Work out the finished part from the listing and answer in its coordinate system (mm). A direction names the side the tool comes from. Give positions to 0.01 mm unless a question says otherwise; leave off trailing zeros. Write each loop counter-clockwise with the first axis right and the second up, starting at its lowest first coordinate (ties: lowest second). Pieces come first, ordered by that corner, then holes. Notation, with made-up numbers: (28, -38.75) - (44, -38.75) arc R27 ccw to (44, -9.75) - close; hole circle Ø1 at (28, -24). An arc over 180 degrees is marked (long way). Write item = value, one per line.
from build123d import *

# Parameters (mm, degrees)
F0_W     = 64
F0_H     = 80
F0_W_2   = 1
F1_DEPTH = 10
F2_T     = -2
F3_DEPTH = 8
F5_DEPTH = 130.001
F6_START = -25.25
F4_R     = 1
F6_DEPTH = 27.25
F8_W     = 1.5
F8_H     = 2
F9_DEPTH = 2.4
F10_R    = 5
F11_R    = 3


# Not quite as in the source:
# - a pattern or mirror of a feature is missing from the dataset's text; its kind, count and spacing are read off the source's solid


with BuildPart() as f1:
    # F0 (on Top) → F1 (new body)
    with BuildSketch(Plane.XY):
        with Locations((-32, 40)):
            Rectangle(F0_W, F0_H)
        with Locations((-64.5, 40)):
            Rectangle(F0_W_2, F0_H)
        with Locations((-65.5, 40)):
            Rectangle(F0_W_2, F0_H)
        with Locations((-98, 40)):
            Rectangle(F0_W, F0_H)
    extrude(amount=F1_DEPTH)

    # F2
    f2_openings = [f1.faces().sort_by_distance(p)[0] for p in [
        (-65, 40, 10),
    ]]
    offset(amount=F2_T, openings=f2_openings)

    # F0 (on Top) → F3 (join)
    with BuildSketch(Plane.XY):
        with Locations((-65.5, 40)):
            Rectangle(F0_W_2, F0_H)
        with Locations((-64.5, 40)):
            Rectangle(F0_W_2, F0_H)
    extrude(amount=F3_DEPTH)

    # F4 (on face) → F5 (cut, through all)
    with BuildSketch(Plane.YZ):
        with BuildLine():
            ThreePointArc((0, 7.8458905733), (0.7245313434, 8.5770948967), (0.9894327009, 9.5717972144))
            ThreePointArc((0.9894327009, 9.5717972144), (0.9778046189, 9.7871506811), (0.9430555853, 10))
            Line((0.9430555853, 10), (0.840551923, 10))
            ThreePointArc((0.840551923, 10), (0.8771729534, 9.7872890681), (0.8894327009, 9.5717972144))
            ThreePointArc((0.8894327009, 9.5717972144), (0.6522733229, 8.6525795765), (0, 7.9628367631))
            Line((0, 7.9628367631), (0, 7.8458905733))
        make_face()
        with BuildLine():
            ThreePointArc((0.8894327009, 9.5717972144), (0.8771729534, 9.7872890681), (0.840551923, 10))
            Line((0.840551923, 10), (0, 10))
            Line((0, 10), (0, 7.9628367631))
            ThreePointArc((0, 7.9628367631), (0.6522733229, 8.6525795765), (0.8894327009, 9.5717972144))
        make_face()
    extrude(amount=-F5_DEPTH, mode=Mode.SUBTRACT)

    # F4 (on face) → F6 (join)
    with BuildSketch(Plane.YZ.offset(F6_START)):
        with BuildLine():
            ThreePointArc((0, 7.8458905733), (0.7245313434, 8.5770948967), (0.9894327009, 9.5717972144))
            ThreePointArc((0.9894327009, 9.5717972144), (0.9778046189, 9.7871506811), (0.9430555853, 10))
            Line((0.9430555853, 10), (0.840551923, 10))
            ThreePointArc((0.840551923, 10), (0.8771729534, 9.7872890681), (0.8894327009, 9.5717972144))
            ThreePointArc((0.8894327009, 9.5717972144), (0.6522733229, 8.6525795765), (0, 7.9628367631))
            Line((0, 7.9628367631), (0, 7.8458905733))
        make_face()
        with BuildLine():
            Line((0.840551923, 10), (0.9430555853, 10))
            ThreePointArc((0.9430555853, 10), (-2.8426843031, 10.3738865383), (0, 7.8458905733))
            Line((0, 7.8458905733), (0, 7.9628367631))
            ThreePointArc((0, 7.9628367631), (-2.7669331351, 10.2964895976), (0.840551923, 10))
        make_face()
        with BuildLine():
            ThreePointArc((0.8894327009, 9.5717972144), (0.8771729534, 9.7872890681), (0.840551923, 10))
            Line((0.840551923, 10), (0, 10))
            Line((0, 10), (0, 7.9628367631))
            ThreePointArc((0, 7.9628367631), (0.6522733229, 8.6525795765), (0.8894327009, 9.5717972144))
        make_face()
        with BuildLine():
            Line((0, 10), (0.840551923, 10))
            ThreePointArc((0.840551923, 10), (-2.7669331351, 10.2964895976), (0, 7.9628367631))
            Line((0, 7.9628367631), (0, 10))
        make_face()
        with Locations((-1.0105672991, 9.5717972144)):
            Circle(F4_R, mode=Mode.SUBTRACT)
    f6 = extrude(amount=-F6_DEPTH)

    # F6_copies: F6 across plane
    add(f6.mirror(Plane(origin=(-65, 0, 0), x_dir=(0, 0, -1), z_dir=(-1, 0, 0))))

    # F8 (on mid) → F9 (join, symmetric)
    with BuildSketch(Plane(origin=(-65, 0, 0), x_dir=(0, -1, 0), z_dir=(-1, 0, 0))):
        Polygon((-80, 13.2), (-80, 11.2), (-78.6, 11.7), (-78.6, 12.7), align=None)
        Polygon((-81.5, 10), (-80, 10), (-80, 11.2), (-80, 13.2), (-81.5, 13.2), align=None)
        with Locations((-80.75, 9)):
            Rectangle(F8_W, F8_H)
    extrude(amount=F9_DEPTH, both=True)

    # F10
    f10_edges = [f1.edges().sort_by_distance(p)[0] for p in [
        (-33, 2, 2),
        (-64, 40, 2),
        (-33, 78, 2),
        (-2, 40, 2),
        (-97, 2, 2),
        (-128, 40, 2),
        (-97, 78, 2),
        (-66, 40, 2),
    ]]
    fillet(f10_edges, radius=F10_R)

    # F11
    f11_edges = [f1.edges().sort_by_distance(p)[0] for p in [
        (-130, 80, 5),
        (0, 80, 5),
    ]]
    fillet(f11_edges, radius=F11_R)


solid = f1.part
1. Find section A-A, the plane x = -85. Give the vertices of the cut face in (y, z).
Solution:
outline = (0, 0) - (80, 0) - (80, 10) - (78, 10) - (78, 7) arc R5 cw to (73, 2) - (7, 2) arc R5 cw to (2, 7) - (2, 10) - (0.94, 10) arc R2 ccw (long way) to (0, 7.85) - close; hole circle Ø2 at (-1.01, 9.57)
2. A tool of negligible diameter and unlimited length cuts with its end or side. For faces 4 (the flat face through (-65, 81.5, 11)), 5 (the flat face through (-33, 40, 2)), 6 (the flat face through (-67.4, 80.4, 11.2)), 7 (the flat face through (-62.6, 80.4, 11.2)), from which of +Z, -Z, +X, -X, +Y, -Y can it reach the whole face along a straight path? Write none if from no direction.
Solution:
face_4 = +Z, -Z, +X, -X, +Y
face_5 = +Z
face_6 = +Z, -X, +Y
face_7 = +Z, +X, +Y
3. Find section C-C, the plane y = 33. Give the vertices of the cut face in (x, z), then the cut area to 3 significant figures.
Solution:
outline = (-130, 0) - (0, 0) - (0, 10) - (-2, 10) - (-2, 7) arc R5 cw to (-7, 2) - (-59, 2) arc R5 cw to (-64, 7) - (-64, 8) - (-66, 8) - (-66, 7) arc R5 cw to (-71, 2) - (-123, 2) arc R5 cw to (-128, 7) - (-128, 10) - (-130, 10) - close
area = 325 mm^2
4. Find section B-B, the plane z = 4.75. Give the vertices of the cut face in (x, y).
Solution:
outline = (-130, 0) - (0, 0) - (0, 77) arc R3 ccw to (-3, 80) - (-127, 80) arc R3 ccw to (-130, 77) - close; hole (-127.47, 2.53) - (-66.53, 2.53) - (-66.53, 77.47) - (-127.47, 77.47) - close; hole (-63.47, 2.53) - (-2.53, 2.53) - (-2.53, 77.47) - (-63.47, 77.47) - close
5. For a pull along Y with two mould halves and no side action, classify faces 1 (the flat face through (-64.1, 78, 8.5)), 2 (the flat face through (-130, 38, 5)), 3 (the cylindrical face through (-0.9, 79.14, 5.07)) as pulls with the +Y half, pulls with the -Y half, needs draft (parallel to the pull), parting line crosses it, or undercut.
Solution:
face_1 = undercut
face_2 = needs draft
face_3 = pulls with the +Y half
6. Find section D-D, the plane x = -20.5. Give the vertices of the cut face in (y, z), then the cut area to 3 significant figures.
Solution:
outline = (0, 0) - (80, 0) - (80, 10) - (78, 10) - (78, 7) arc R5 cw to (73, 2) - (7, 2) arc R5 cw to (2, 7) - (2, 10) - (0.94, 10) arc R2 cw to (0, 7.85) - close
area = 201 mm^2
7. Straight lines are drawn through the part: line 1 (Y direction, x = -52, z = 9.75); line 2 (X direction, y = 54, z = 7.25); line 3 (X direction, y = 9.5, z = 8.5). For each, find the intervals that lie inside material, in ascending order.
Solution:
line_1 = -3 to -1.99, -0.03 to 2, 78 to 80
line_2 = -130 to -128, -66 to -64, -2 to 0
line_3 = -130 to -128, -2 to 0
8. Given pin 1 (23.5 mm diameter, centred on x = -71.5, y = 26, fed in from +Z); pin 2 (2 mm diameter, centred on y = -1.5, z = 9.5, fed in from +X); pin 3 (1.5 mm diameter, centred on x = -25.5, y = 56, fed in from +Z), each flat-ended and moving along its own axis, determine where each tip first touches the part or whether it passes through.
Solution:
pin_1 = 8
pin_2 = -25.25
pin_3 = 2
